Here's how the part is built. I have some questions about the finished solid (model axes, mm). A direction names the side the tool comes from. Coordinates: 2 decimals unless noted, no trailing zeros. Write each loop counter-clockwise with the first axis right and the second up, starting at its lowest first coordinate (ties: lowest second). Pieces come first, ordered by that corner, then holes. Notation, with made-up numbers: (-34, -35) -> (3, -35) arc R20 ccw to (3, -22) -> close; hole circle Ø1 at (-21, 87.25). An arc over 180 degrees is marked (long way). Use a Markdown table: item, result. Add a question column.
Item 1: On a 3-axis mill with a long thin cutter (end or side, diameter ignored), from which of +Z, -Z, +X, -X, +Y, -Y can I reach the whole of each face in a straight line? I mean faces 5 (the cylindrical face through (-2.579, -1.978, 4.056)), 6 (the flat face through (-6, 0, 1)), 7 (the flat face through (0, 0, -8)), 8 (the flat face through (18, 0, -6)), 9 (the flat face through (6, 0, 1)). Say none if no direction works.
Item 2: Imagine slicing it at C-C, the plane z = 4.75. Write out the boundary of the cut face in (x, y), and give its area (3 significant figures).
Item 3: If I drill on line 1 along Y through (x, z) = (0, 6.25); line 2 along Y through (x, z) = (12, -6.3); line 3 along Z through (x, y) = (2.5, 0.75), over which ranges is the centre line in solid material (lowest first)? Write a range as from..to.
Item 4: Imagine slicing it at A-A, the plane y = 0. Write out the boundary of the cut face in (x, z), and give its area (3 significant figures).
Item 5: Will these pins go through, and if not, where does the flat tip stop? pin 1 Ø8 at (x, z) = (10.5, -0.5) entering from +Y; pin 2 Ø6.5 at (x, y) = (12, 0) entering from +Z; pin 3 Ø4 at (y, z) = (-3, 0) entering from +X.
Item 6: Imagine slicing it at D-D, the plane x = 0. Write out the boundary of the cut face in (y, z).
Item 7: Imagine slicing it at B-B, the plane x = 12. Write out the boundary of the cut face in (y, z).
Item 8: If we mould it in two halves opening along Y, with no side actions, what happens to faces 1 (the cylindrical face through (13.6, 1.2, -6.5)), 2 (the flat face through (0, -6, -2)), 3 (the flat face through (3, 3, 8)), 4 (the flat face through (0, 6, -2))? For each: pulls with the +Y half, pulls with the -Y half, needs draft (parallel to the pull), parting line crosses it, or undercut.
```python
from build123d import *

# Parameters (mm, degrees)
CROQUIS1_W              = 36
CROQUIS1_H              = 12
SALIENTE_EXTRUIR1_DEPTH = 8
CROQUIS2_R              = 3.25
CORTAR_EXTRUIR1_DEPTH   = 8
CROQUIS3_W              = 12
CROQUIS3_H              = 13
CORTAR_EXTRUIR2_DEPTH   = 24.065125189
CROQUIS4_R              = 2
CORTAR_EXTRUIR3_DEPTH   = 8


with BuildPart() as part:
    # Croquis1 → Saliente-Extruir1 (new, symmetric)
    with BuildSketch(Plane.XY):
        Rectangle(CROQUIS1_W, CROQUIS1_H)
    extrude(amount=SALIENTE_EXTRUIR1_DEPTH, both=True)

    # Croquis2 → Cortar-Extruir1 (cut)
    with BuildSketch(Plane.XY.offset(8)):
        Circle(CROQUIS2_R)
    extrude(amount=-CORTAR_EXTRUIR1_DEPTH, mode=Mode.SUBTRACT)

    # Croquis3 → Cortar-Extruir2 (cut, through all)
    with BuildSketch(Plane.XZ.offset(6)):
        with Locations((-12, 1.5)):
            Rectangle(CROQUIS3_W, CROQUIS3_H)
        with Locations((12, 1.5)):
            Rectangle(CROQUIS3_W, CROQUIS3_H)
    extrude(amount=-CORTAR_EXTRUIR2_DEPTH, mode=Mode.SUBTRACT)

    # Croquis4 → Cortar-Extruir3 (cut)
    with BuildSketch(Plane.XY.offset(-5)):
        with Locations((-12, 0)):
            Circle(CROQUIS4_R)
        with Locations(Location((12, 0, 0), (0, 0, 180))):
            Circle(CROQUIS4_R)
    extrude(amount=-CORTAR_EXTRUIR3_DEPTH, mode=Mode.SUBTRACT)


solid = part.part
```
Ans:
| question | item | result |
|---|---|---|
| 1 | face 5 | +Z |
| 1 | face 6 | +Z, -X, +Y, -Y |
| 1 | face 7 | -Z, +X, -X, +Y, -Y |
| 1 | face 8 | +Z, -Z, +X, +Y, -Y |
| 1 | face 9 | +Z, +X, +Y, -Y |
| 2 | outline | (-6, -6) -> (6, -6) -> (6, 6) -> (-6, 6) -> close; hole circle Ø6.5 at (0, 0) |
| 2 | area | 111 mm^2 |
| 3 | line 1 | y = -6..-3.25, 3.25..6 |
| 3 | line 2 | y = -6..-2, 2..6 |
| 3 | line 3 | z = -8..0 |
| 4 | outline | (-18, -8) -> (-14, -8) -> (-14, -5) -> (-18, -5) -> close; (-10, -8) -> (10, -8) -> (10, -5) -> (6, -5) -> (6, 8) -> (3.25, 8) -> (3.25, 0) -> (-3.25, 0) -> (-3.25, 8) -> (-6, 8) -> (-6, -5) -> (-10, -5) -> close; (14, -8) -> (18, -8) -> (18, -5) -> (14, -5) -> close |
| 4 | area | 188 mm^2 |
| 5 | pin 1 | passes through |
| 5 | pin 2 | stops at z = -5 |
| 5 | pin 3 | stops at x = 6 |
| 6 | outline | (-6, -8) -> (6, -8) -> (6, 8) -> (3.25, 8) -> (3.25, 0) -> (-3.25, 0) -> (-3.25, 8) -> (-6, 8) -> close |
| 7 | outline | (-6, -8) -> (-2, -8) -> (-2, -5) -> (-6, -5) -> close; (2, -8) -> (6, -8) -> (6, -5) -> (2, -5) -> close |
| 8 | face 1 | undercut |
| 8 | face 2 | pulls with the -Y half |
| 8 | face 3 | needs draft |
| 8 | face 4 | pulls with the +Y half |
